from build123d import *

# Parameters (mm, degrees)
SKETCH_2_R          = 1.2
CUT_EXTRUDE_1_DEPTH = 10
SKETCH_3_R          = 2.475
CUT_EXTRUDE_2_DEPTH = 3
SKETCH_4_R          = 1
CUT_EXTRUDE_3_DEPTH = 3


with BuildPart() as part:
    # 草图1 → 旋转1 (revolve)
    with BuildSketch(Plane.XY, mode=Mode.PRIVATE) as revolve_1_sk:
        Polygon((0, 0), (10, 0), (10, 2.5), (3.75, 2.5), (3.75, 4.5), (0, 4.5), align=None)
    revolve(revolve_1_sk.sketch.rotate(Axis((0, 0, 0), (0, 1, 0)), 90), axis=Axis((0, 0, 0), (0, 1, 0)))

    # 草图2 → 切除-拉伸1 (cut)
    with BuildSketch(Plane(origin=(0, 4.5, 0), x_dir=(1, 0, 0), z_dir=(0, 1, 0))):
        with Locations(Location((0, 0, 0), (0, 0, 270))):
            Circle(SKETCH_2_R)
    extrude(amount=-CUT_EXTRUDE_1_DEPTH, mode=Mode.SUBTRACT)

    # 草图3 → 切除-拉伸2 (cut)
    with BuildSketch(Plane(origin=(0, 4.5, 0), x_dir=(1, 0, 0), z_dir=(0, 1, 0))):
        with Locations(Location((0, 0, 0), (0, 0, 270))):
            Circle(SKETCH_3_R)
    extrude(amount=-CUT_EXTRUDE_2_DEPTH, mode=Mode.SUBTRACT)

    # 草图4 → 切除-拉伸3 (cut)
    with BuildSketch(Plane.XZ):
        with Locations(Location((7, 0, 0), (0, 0, 270))):
            Circle(SKETCH_4_R)
        with Locations(Location((0, -7, 0), (0, 0, 270))):
            Circle(SKETCH_4_R)
        with Locations(Location((-7, 0, 0), (0, 0, 270))):
            Circle(SKETCH_4_R)
        with Locations(Location((0, 7, 0), (0, 0, 270))):
            Circle(SKETCH_4_R)
    extrude(amount=-CUT_EXTRUDE_3_DEPTH, mode=Mode.SUBTRACT)


solid = part.part
Model file for the job. Use its own axes, mm. A direction names the side the tool comes from. Round coordinates to 2 decimals unless told otherwise and drop trailing zeros. Loops run counter-clockwise (first coordinate to the right, second up) from the corner with the lowest first, then second, coordinate; pieces in that order, holes last. Notation, with made-up numbers: M -12,33 L 32,33 A23 ccw 32,42 Z; hole C -9,30 d9. An arc over 180 degrees is marked long. One line per question, with ' | ' between items.
1) Band-saw the part on B-B (x = 0). Give the cut face in (y, z) (3 decimals).
Solved:
outline: M 0,-10 L 2.5,-10 L 2.5,-8 L 0,-8 Z; M 0,-6 L 2.5,-6 L 2.5,-3.75 L 4.5,-3.75 L 4.5,-2.475 L 1.5,-2.475 L 1.5,-1.2 L 0,-1.2 Z; M 0,1.2 L 1.5,1.2 L 1.5,2.475 L 4.5,2.475 L 4.5,3.75 L 2.5,3.75 L 2.5,6 L 0,6 Z; M 0,8 L 2.5,8 L 2.5,10 L 0,10 Z
2) Mould opens along X. For faces 3 (the cylindrical face through (-3.16, 3.51, -2.02)), 4 (the cylindrical face through (-0.6, 1.2, 7.8)), 5 (the cylindrical face through (-0.6, 1.2, -6.2)), 6 (the flat face through (2, 0, 0)) say: +X half, -X half, draft (parallel to the pull), parting line (faces both ways), or undercut.
Solved:
face 3: parting line | face 4: undercut | face 5: undercut | face 6: draft
3) Band-saw the part on D-D (z = -7). Give the cut face in (x, y).
Solved:
outline: M -7.14,0 L -1,0 L -1,2.5 L -7.14,2.5 Z; M 1,0 L 7.14,0 L 7.14,2.5 L 1,2.5 Z
4) Band-saw the part on C-C (x = -7). Give the cut face in (y, z), then the cut area to 3 significant figures.
Solved:
outline: M 0,-7.14 L 2.5,-7.14 L 2.5,-1 L 0,-1 Z; M 0,1 L 2.5,1 L 2.5,7.14 L 0,7.14 Z | area: 30.7 mm²
5) Band-saw the part on A-A (z = 0). Give the cut face in (x, y) (3 decimals).
Solved:
outline: M -10,0 L -8,0 L -8,2.5 L -10,2.5 Z; M -6,0 L -1.2,0 L -1.2,1.5 L -2.475,1.5 L -2.475,4.5 L -3.75,4.5 L -3.75,2.5 L -6,2.5 Z; M 1.2,0 L 6,0 L 6,2.5 L 3.75,2.5 L 3.75,4.5 L 2.475,4.5 L 2.475,1.5 L 1.2,1.5 Z; M 8,0 L 10,0 L 10,2.5 L 8,2.5 Z
6) Flat gauge pins, fed straight in: pin 1 (2.5 mm diameter, centred on x = -7, z = 0, fed in from +Y); pin 2 (3 mm diameter, centred on x = 0, z = 0, fed in from -Y); pin 3 (1 mm diameter, centred on y = 4, z = 0.5, fed in from +X); pin 4 (3 mm diameter, centred on x = 0, z = 0, fed in from +Y). Where does each tip first touch, or does it go through?
Solved:
pin 1: stops at y = 2.5 | pin 2: stops at y = 0 | pin 3: stops at x = 3.75 | pin 4: stops at y = 1.5
7) 3-axis set-ups, long thin cutter, end or side, ignore diameter. For faces 1 (the cylindrical face through (0.74, 3.02, 2.36)), 2 (the flat face through (-3, 4.5, 0)): which of +Z, -Z, +X, -X, +Y, -Y reach the whole face in a straight line?
Solved:
face 1: +Y | face 2: +Z, -Z, +X, -X, +Y
8) Drill centre lines: line 1 along X through (y, z) = (2.05, 0) (3 decimals); line 2 along X through (y, z) = (1.3, 0); line 3 along Z through (x, y) = (0.25, 0.6). Where is each one in solid material? Low to high.
Solved:
line 1: x = -10 to -8, -6 to -2.475, 2.475 to 6, 8 to 10 | line 2: x = -10 to -8, -6 to -1.2, 1.2 to 6, 8 to 10 | line 3: z = -10 to -7.97, -6.03 to -1.17, 1.17 to 6.03, 7.97 to 10
